Autodesk Inventor part; units mm, degrees
ref_plane "YZ Plane" through (0, 0, 0) normal (1, 0, 0) x (0, 1, 0)
ref_plane "XZ Plane" through (0, 0, 0) normal (0, 1, 0) x (-1, 0, 0)
ref_plane "XY Plane" through (0, 0, 0) normal (0, 0, 1) x (1, 0, 0)
sketch "Эскиз1" plane through (0, 0, 0) normal (0, 0, 1) x (1, 0, 0)
  line L0 (-177.5, -105) -> (177.5, -105)
  line L1 (177.5, -105) -> (177.5, 105)
  line L2 (177.5, 105) -> (-177.5, 105)
  line L3 (-177.5, 105) -> (-177.5, -105)
  line L4 (-177.5, -105) -> (177.5, 105) construction
  line L5 (177.5, -105) -> (-177.5, 105) construction
  point P0 (0, 0)
  dimension "d0" = 355
  dimension "d1" = 210
extrude "Выдавливание1" add sketch "Эскиз1" along normal blind 4
sketch "Эскиз2" plane through (0, 0, 4) normal (0, 0, 1) x (1, 0, 0)
  line L0 (-177.5, 105) -> (-177.5, -105)
  line L1 (177.5, -105) -> (177.5, 105)
  line L2 (-177.5, -105) -> (177.5, -105)
  line L3 (177.5, -105) -> (177.5, -30)
  line L4 (177.5, -30) -> (-177.5, -30)
  line L5 (-177.5, -30) -> (-177.5, -105)
  line L6 (177.5, 105) -> (-177.5, 105)
  point P0 (0, 0)
  dimension "d4" = 135
extrude "Выдавливание2" add sketch "Эскиз2" along normal blind 4 contours L4 L1 L2 L0
properties part number "монитор"
The model under review builds one solid part; all positions refer to its coordinate system, in mm. A direction names the side the tool comes from. Round coordinates to 2 decimals unless told otherwise and drop trailing zeros. Loops run counter-clockwise (first coordinate to the right, second up) from the corner with the lowest first, then second, coordinate; pieces in that order, holes last.
Item 1: For line 1 (Z direction, x = 9.5, y = 53); line 2 (Y direction, x = 127, z = 5.5), list the stretches that pass through material, from the lowest coordinate up.
Determined:
line 1: z = 0 to 4
line 2: y = -105 to -30
Item 2: For faces 1 (the face through (-2, 1, 0)), 2 (the face through (-2, 38, 4)), list the 3-axis set-ups (+Z, -Z, +X, -X, +Y, -Y) from which the entire face can be reached by the end or side of a thin tool; tool diameter is ignored.
Determined:
face 1: -Z, +X, -X, +Y, -Y
face 2: +Z, +X, -X, +Y
Item 3: Take a section at A-A (x = -21.5). Write out the cut boundary in (y, z).
Determined:
outline: (-105, 0) - (105, 0) - (105, 4) - (-30, 4) - (-30, 8) - (-105, 8) - close
Item 4: Clearance check with flat-ended pins moving along their axes: pin 1 Ø8 at (x, y) = (54, -34) entering from -Z; pin 2 Ø1.5 at (x, z) = (49, 5.5) entering from +Y. State where each tip first meets the part, or that it passes through.
Determined:
pin 1: stops at z = 0
pin 2: stops at y = -30
Item 5: Take a section at C-C (z = 5.5). Write out the cut boundary in (x, y).
Determined:
outline: (-177.5, -105) - (177.5, -105) - (177.5, -30) - (-177.5, -30) - close
Item 6: Take a section at B-B (y = 62.5). Write out the cut boundary in (x, z), then the cut area to 3 significant figures.
Determined:
outline: (-177.5, 0) - (177.5, 0) - (177.5, 4) - (-177.5, 4) - close
area: 1,420 mm2
